from build123d import *

# Parameters (mm, degrees)
F1_DEPTH = 20
F3_R     = 3.6
F4_DEPTH = 20.001
F2_R     = 3.6
F5_DEPTH = 20.001
F6_START = -3.5
F3_R_2   = 5.5
F6_DEPTH = 16.501
F7_START = -3.5
F2_R_2   = 5.5
F7_DEPTH = 16.501


with BuildPart() as f1:
    # F0 (on Front) → F1 (new body)
    with BuildSketch(Plane.XZ):
        Polygon((-13.2217891409, 3.8167946823), (-13.2217891409, 2.8167946823), (6.7782108591, 2.8167946823), (6.7782108591, 22.8167946823), (5.7782108591, 22.8167946823), align=None)
    extrude(amount=F1_DEPTH)

    # F3 (on face) → F4 (cut, through all)
    with BuildSketch(Plane.YZ.offset(6.7782108591)):
        with Locations((-10, 12.8167946823)):
            Circle(F3_R)
    extrude(amount=-F4_DEPTH, mode=Mode.SUBTRACT)

    # F2 (on face) → F5 (cut, through all)
    with BuildSketch(Plane(origin=(0, 0, 2.8167946823), x_dir=(1, 0, 0), z_dir=(0, 0, -1))):
        with Locations((-3.2217891409, 10)):
            Circle(F2_R)
    extrude(amount=-F5_DEPTH, mode=Mode.SUBTRACT)

    # F3 (on face) → F6 (cut)
    with BuildSketch(Plane.YZ.offset(6.7782108591).offset(F6_START)):
        with Locations((-10, 12.8167946823)):
            Circle(F3_R_2)
        with Locations((-10, 12.8167946823)):
            Circle(F3_R, mode=Mode.SUBTRACT)
    extrude(amount=-F6_DEPTH, mode=Mode.SUBTRACT)

    # F2 (on face) → F7 (cut)
    with BuildSketch(Plane(origin=(0, 0, 2.8167946823), x_dir=(1, 0, 0), z_dir=(0, 0, -1)).offset(F7_START)):
        with Locations((-3.2217891409, 10)):
            Circle(F2_R_2)
        with Locations((-3.2217891409, 10)):
            Circle(F2_R, mode=Mode.SUBTRACT)
    extrude(amount=-F7_DEPTH, mode=Mode.SUBTRACT)


solid = f1.part
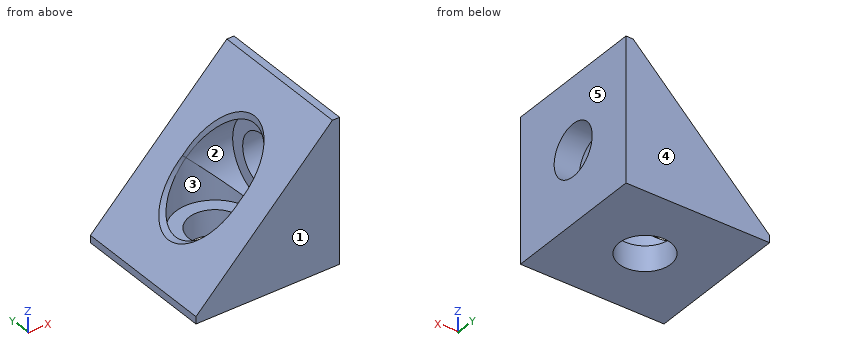
Read the model definition and answer for the solid it produces. Units are mm, in the model's axes. Face numbers are marked on the shaded views. A direction names the side the tool comes from. Coordinates: 2 decimals unless noted, no trailing zeros. Write each loop counter-clockwise with the first axis right and the second up, starting at its lowest first coordinate (ties: lowest second). Pieces come first, ordered by that corner, then holes. Notation, with made-up numbers: (-4.75, 79.5) - (21.25, 79.5) arc R23 cw to (21.25, 99.5) - close; hole circle Ø6 at (-13, 15.5). An arc over 180 degrees is marked (long way). One line per question, with ' | ' between items.
Q1. For the marked faces 1 and 2, determine the directions among +Z, -Z, +X, -X, +Y, -Y from which every point of the face is accessible in a straight line to the end or side of a thin tool.
Result set:
face 1: +Z, -Z, +X, -X, -Y | face 2: -X
Q2. Find section B-B, the plane z = 9.75. Write down the section's boundary in (x, y) (3 decimals).
Result set:
outline: (-7.289, -20) - (6.778, -20) - (6.778, -11.885) - (3.278, -11.885) - (3.278, -14.566) - (-0.155, -14.566) arc R5.5 cw to (-6.289, -14.566) - (-7.289, -14.566) - close; (-7.289, -5.434) - (-6.289, -5.434) arc R5.5 cw to (-0.155, -5.434) - (3.278, -5.434) - (3.278, -8.115) - (6.778, -8.115) - (6.778, 0) - (-7.289, 0) - close
Q3. Find section D-D, the plane z = 16.75. Write down the section's boundary in (x, y).
Result set:
outline: (-0.29, -20) - (6.78, -20) - (6.78, 0) - (-0.29, 0) - (-0.29, -5.35) arc R5.5 cw to (0.71, -6.16) - (3.28, -6.16) - (3.28, -13.84) - (0.71, -13.84) arc R5.5 cw to (-0.29, -14.65) - close
Q4. Consider L1, parallel to X at y = -11.75, z = 8; L2, parallel to Z at x = 2.5, y = -10.5; L3, parallel to Z at x = 5.1, y = -10. Determine where each line is inside the solid, lowest interval first. Write a range as [from, to].
Result set:
L1: [3.28, 6.78] | L2: [2.82, 7.34], [18.29, 19.54] | L3: [2.82, 9.22], [16.42, 22.14]
Q5. Determine the mould class of the marked faces 3, 4 and 5 for opening direction Y: +Y half, -Y half, draft (parallel to the pull), parting line (faces both ways), or undercut.
Result set:
face 3: undercut | face 4: +Y half | face 5: draft
Q6. Each of these flat-tipped pins is pushed along its axis until it touches: P1, Ø9.5, axis at y = -10, z = 12.82, coming from the -X side; P2, Ø6.5, axis at x = -3.22, y = -10, coming from the +Z side; P3, Ø12, axis at x = -0.5, y = -10.5, coming from the +Z side; P4, Ø9, axis at x = -3.22, y = -10, coming from the -Z side. Where does it stop, or does it pass through?
Result set:
P1: x = 3.28 | P2: through | P3: z = 22.54 | P4: z = 2.82
Q7. Find section C-C, the plane x = -1.5. Write down the section's boundary in (y, z) (3 decimals).
Result set:
outline: (-20, 2.817) - (-13.162, 2.817) - (-13.162, 6.317) - (-15.224, 6.317) - (-15.224, 11.095) arc R5.5 cw to (-15.224, 14.539) - (-15.224, 15.539) - (-20, 15.539) - close; (-6.838, 2.817) - (0, 2.817) - (0, 15.539) - (-4.776, 15.539) - (-4.776, 14.539) arc R5.5 cw to (-4.776, 11.095) - (-4.776, 6.317) - (-6.838, 6.317) - close
Q8. Find section A-A, the plane y = -10. Write down the section's boundary in (x, z).
Result set:
outline: (-13.22, 2.82) - (-6.82, 2.82) - (-6.82, 6.32) - (-8.72, 6.32) - (-8.72, 7.32) - (-9.72, 7.32) - (-13.22, 3.82) - close; (0.38, 2.82) - (6.78, 2.82) - (6.78, 9.22) - (3.28, 9.22) - (3.28, 7.32) - (2.28, 7.32) - (2.28, 6.32) - (0.38, 6.32) - close; (2.28, 18.32) - (3.28, 18.32) - (3.28, 16.42) - (6.78, 16.42) - (6.78, 22.82) - (5.78, 22.82) - (2.28, 19.32) - close
